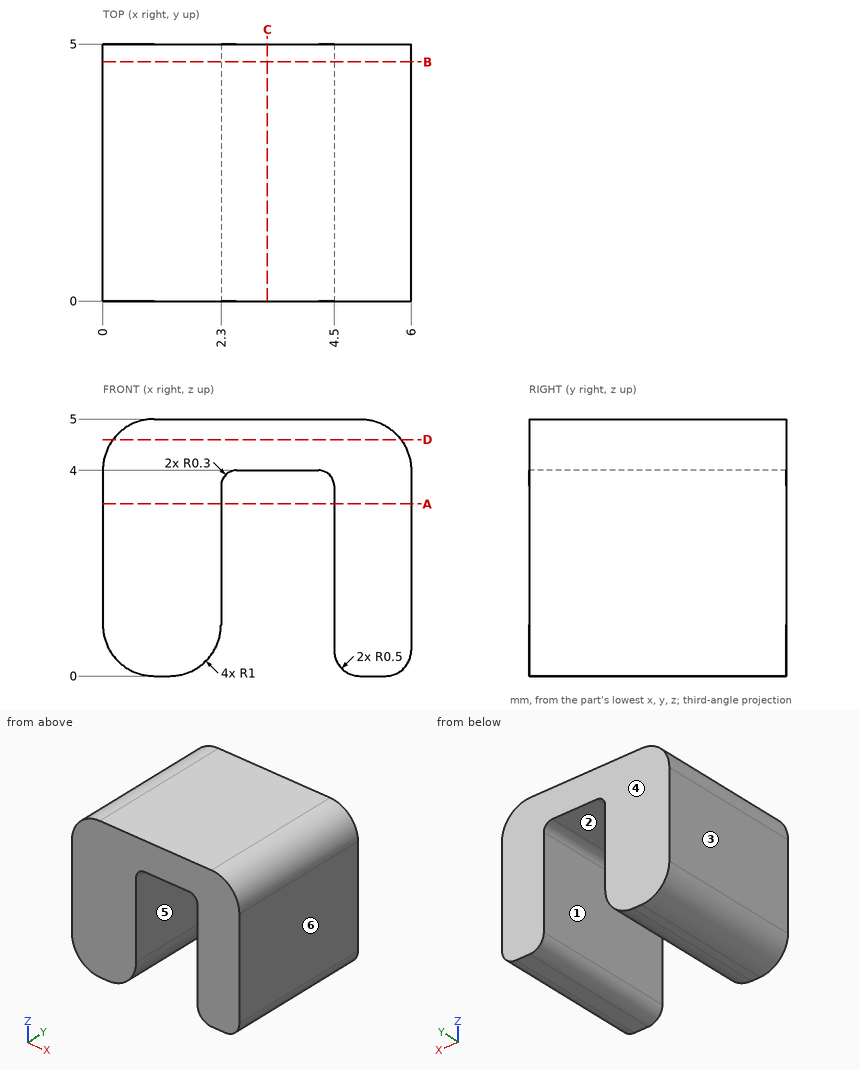
Here's the drawing with two shaded views (mm, measured from the low corner). I have some questions. A direction names the side the tool comes from. Coordinates: 2 decimals unless noted, no trailing zeros. Order: outer loops, then holes, each group sorted by start corner. A loop starts at its lowest first (then second) coordinate and runs counter-clockwise, first axis right, second up. Notation, with made-up numbers: M 0,-24 L 43,-24 A8 ccw 43,-13 Z; hole C -37,52.5 d5. An arc over 180 degrees is marked long. Write item = value, one per line.
(1) Suppose I cut it at D-D on z = 4.6. Please give me the cut outline in (x, y), plus the area to 3 significant figures.
Results are:
outline = M 0.2,0 L 5.8,0 L 5.8,5 L 0.2,5 Z
area = 28.0 mm2
(2) For the marked faces 5 and 6, which set-ups out of +Z, -Z, +X, -X, +Y, -Y let a thin tool reach every point of the face, with its end or its side?
Results are:
face_5 = -Z, +Y, -Y
face_6 = +Z, -Z, +X, +Y, -Y
(3) Suppose I cut it at B-B on y = 4.65. Please give me the cut outline in (x, z), plus the area to 3 significant figures.
Results are:
outline = M 0,1 A1 ccw 1,0 L 1.3,0 A1 ccw 2.3,1 L 2.3,3.7 A0.3 cw 2.6,4 L 4.2,4 A0.3 cw 4.5,3.7 L 4.5,0.5 A0.5 ccw 5,0 L 5.5,0 A0.5 ccw 6,0.5 L 6,4 A1 ccw 5,5 L 1,5 A1 ccw 0,4 Z
area = 20.3 mm2
(4) Suppose I cut it at C-C on x = 3.2. Please give me the cut outline in (y, z).
Results are:
outline = M 0,4 L 5,4 L 5,5 L 0,5 Z
(5) If we mould it in two halves opening along X, with no side actions, what happens to the marked faces 1, 2, 3 and 4? For each: pulls with the +X half, pulls with the -X half, needs draft (parallel to the pull), parting line crosses it, or undercut.
Results are:
face_1 = undercut
face_2 = undercut
face_3 = pulls with the -X half
face_4 = needs draft
(6) For pin 1 Ø0.5 at (x, y) = (3, 2.5) entering from -Z; pin 2 Ø2 at (x, y) = (0.5, 0.5) entering from -Z, each with a flat end and sliding along its axis, tell me the tip position at first contact or that it passes through.
Results are:
pin_1 = 4
pin_2 = 0
(7) Suppose I cut it at A-A on z = 3.35. Please give me the cut outline in (x, y).
Results are:
outline = M 0,0 L 2.3,0 L 2.3,5 L 0,5 Z; M 4.5,0 L 6,0 L 6,5 L 4.5,5 Z
(8) I need wall thicknesses on line 1 along X through (y, z) = (1.4, 3.4); line 2 along X through (y, z) = (4, 0.6); line 3 along Z through (x, y) = (3.7, 2.75). Which ranges of each line are inside material? Lowest first, please. Write a range as [from, to].
Results are:
line_1 = [0, 2.3], [4.5, 6]
line_2 = [0.08, 2.22], [4.5, 6]
line_3 = [4, 5]
